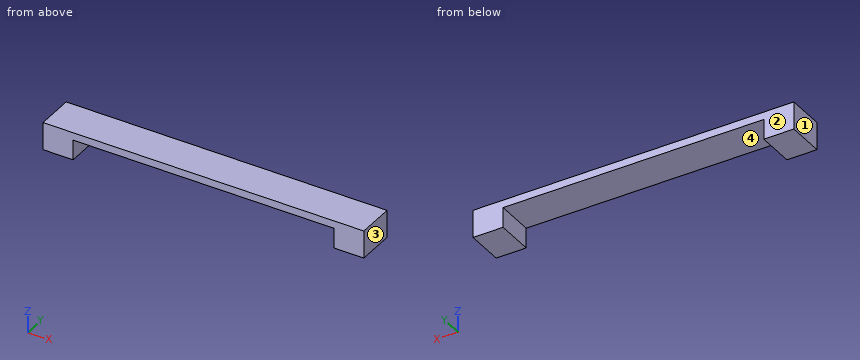
from build123d import *

# Parameters (mm, degrees)
BOX501_W     = 128
BOX501_H     = 15
BOX501_DEPTH = 3
BOX502_W     = 12
BOX502_H     = 15
BOX502_DEPTH = 11
BOX503_W     = 12
BOX503_H     = 15
BOX503_DEPTH = 11


with BuildPart() as box501:
    # Box501 → Box501 (new body)
    with BuildSketch(Plane(origin=(-98, -27, 48), x_dir=(1, 0, 0), z_dir=(0, 0, 1))):
        with Locations((64, 7.5)):
            Rectangle(BOX501_W, BOX501_H)
    extrude(amount=BOX501_DEPTH)


with BuildPart() as box502:
    # Box502 → Box502 (new body)
    with BuildSketch(Plane(origin=(-98, -27, 40), x_dir=(1, 0, 0), z_dir=(0, 0, 1))):
        with Locations((6, 7.5)):
            Rectangle(BOX502_W, BOX502_H)
    extrude(amount=BOX502_DEPTH)


with BuildPart() as fusion392:
    # Box503 → Box503 (new body)
    with BuildSketch(Plane(origin=(18, -27, 40), x_dir=(1, 0, 0), z_dir=(0, 0, 1))):
        with Locations((6, 7.5)):
            Rectangle(BOX503_W, BOX503_H)
    extrude(amount=BOX503_DEPTH)

    # Fusion392: union Box501, Box502
    add(box501.part)
    add(box502.part)


with BuildPart() as fusion392_1:
    # Fusion392 placement: moved
    add(fusion392.part.moved(Location((0, 26, 0))))


solid = fusion392_1.part
Can you work these out from the model? Positions are in its coordinate system, mm. Face numbers are marked on the shaded views. Round coordinates to 2 decimals unless told otherwise and drop trailing zeros. Loops run counter-clockwise (first coordinate to the right, second up) from the corner with the lowest first, then second, coordinate; pieces in that order, holes last. Notation, with made-up numbers: (31.25, -36) - (86.25, -36) arc R19 cw to (86.25, -32) - close; hole circle Ø1 at (73, -11.5). An arc over 180 degrees is marked (long way). Answer in a Markdown table with one row per item. Add a question column.
Q1. I want a section at A-A on z = 44. List the corners of the cut face in (x, y) for me.
Q2. I want a section at B-B on y = 6.5. List the corners of the cut face in (x, z) for me.
Q3. We'd pull the mould along X, two halves only. Please class the marked faces 1, 2, 3 and 4: pulls with the +X half, pulls with the -X half, needs draft (parallel to the pull), parting line crosses it, or undercut.
Q4. For pin 1 Ø1.5 at (x, y) = (-25, 9.5) entering from -Z; pin 2 Ø6 at (x, z) = (-37.5, 44) entering from +Y, each with a flat end and sliding along its axis, tell me the tip position at first contact or that it passes through.
Q5. I want a section at C-C on x = -55. List the corners of the cut face in (y, z) for me.
Q6. I need wall thicknesses on L1, parallel to X at y = 7.25, z = 47.5; L2, parallel to Z at x = 0.5, y = 2.25. Which ranges of each line are inside material? Lowest first, please.
A:
| question | item | result |
|---|---|---|
| 1 | outline | (-98, -1) - (-86, -1) - (-86, 14) - (-98, 14) - close; (18, -1) - (30, -1) - (30, 14) - (18, 14) - close |
| 2 | outline | (-98, 40) - (-86, 40) - (-86, 48) - (18, 48) - (18, 40) - (30, 40) - (30, 51) - (-98, 51) - close |
| 3 | face 1 | pulls with the -X half |
| 3 | face 2 | needs draft |
| 3 | face 3 | pulls with the +X half |
| 3 | face 4 | undercut |
| 4 | pin 1 | z = 48 |
| 4 | pin 2 | through |
| 5 | outline | (-1, 48) - (14, 48) - (14, 51) - (-1, 51) - close |
| 6 | L1 | -98 to -86, 18 to 30 |
| 6 | L2 | 48 to 51 |
